from build123d import *

# Parameters (mm, degrees)
SKETCH1_W              = 44.45
SKETCH1_H              = 76.2
BOSS_EXTRUDE1_DEPTH    = 114.3
CUT_EXTRUDE1_REACH     = 124.516
SKETCH2_R              = 9.525
SKETCH3_W              = 22.86
SKETCH3_H              = 27.94
CUT_EXTRUDE2_DEPTH     = 19.05
CUT_EXTRUDE3_REACH     = 124.516
SKETCH4_W              = 34.925
SKETCH4_H              = 19.05
FILLET1_R              = 9.525
F_10_CLEARANCE_HOLE1_D = 5.1054
CUT_EXTRUDE4_REACH     = 130.421


with BuildPart() as part:
    # Sketch1 → Boss-Extrude1 (new body)
    with BuildSketch(Plane(origin=(0, 0, 0), x_dir=(0, 0, -1), z_dir=(1, 0, 0))):
        Rectangle(SKETCH1_W, SKETCH1_H)
    extrude(amount=BOSS_EXTRUDE1_DEPTH)

    # Sketch2 → Cut-Extrude1 (cut, up to next)
    with BuildSketch(Plane(origin=(114.3, 0, 0), x_dir=(0, 0, -1), z_dir=(1, 0, 0)), mode=Mode.PRIVATE) as cut_extrude1_sk1:
        with Locations((1.588, -4.0132)):
            Circle(SKETCH2_R)
    cut_extrude1_tool1 = extrude(cut_extrude1_sk1.sketch, amount=-CUT_EXTRUDE1_REACH, mode=Mode.PRIVATE) & part.part
    add(cut_extrude1_tool1.solids().sort_by_distance((114.3, -4.0132, -1.588))[0], mode=Mode.SUBTRACT)

    # Sketch3 → Cut-Extrude2 (cut)
    with BuildSketch(Plane.XY.offset(22.225)):
        with Locations((102.87, 24.13)):
            Rectangle(SKETCH3_W, SKETCH3_H)
    extrude(amount=-CUT_EXTRUDE2_DEPTH, mode=Mode.SUBTRACT)

    # Sketch4 → Cut-Extrude3 (cut, up to next)
    with BuildSketch(Plane(origin=(0, 0, 0), x_dir=(0, 0, -1), z_dir=(1, 0, 0)), mode=Mode.PRIVATE) as cut_extrude3_sk1:
        with Locations((4.7625, 28.575)):
            Rectangle(SKETCH4_W, SKETCH4_H)
    cut_extrude3_tool1 = extrude(cut_extrude3_sk1.sketch, amount=CUT_EXTRUDE3_REACH, mode=Mode.PRIVATE) & part.part
    add(cut_extrude3_tool1.solids().sort_by_distance((0, 28.575, -4.7625))[0], mode=Mode.SUBTRACT)

    # Fillet1
    fillet1_edges = [part.edges().sort_by_distance(p)[0] for p in [
        (91.44, 14.605, 3.175),
    ]]
    fillet(fillet1_edges, radius=FILLET1_R)

    # #10 Clearance Hole1 (through all)
    with Locations(Plane(origin=(0, 0, -22.225), x_dir=(-1, 0, 0), z_dir=(0, 0, -1))):
        with Locations((-47.625, 28.6385), (-79.375, -31.8135), (-47.625, -31.8135), (-79.375, 28.6385)):
            Hole(F_10_CLEARANCE_HOLE1_D / 2)

    # Sketch9 → Cut-Extrude4 (cut, up to next)
    with BuildSketch(Plane.XY.offset(22.225), mode=Mode.PRIVATE) as cut_extrude4_sk1:
        with BuildLine():
            Line((50.1777, 28.6385), (50.1777, 26.0985))
            ThreePointArc((50.1777, 26.0985), (47.625, 23.5458), (45.0723, 26.0985))
            Line((45.0723, 26.0985), (45.0723, 28.6385))
            ThreePointArc((45.0723, 28.6385), (47.625, 31.1912), (50.1777, 28.6385))
        make_face()
    cut_extrude4_tool1 = extrude(cut_extrude4_sk1.sketch, amount=-CUT_EXTRUDE4_REACH, mode=Mode.PRIVATE) & part.part
    # Sketch9 → Cut-Extrude4 (cut, up to next)
    with BuildSketch(Plane.XY.offset(22.225), mode=Mode.PRIVATE) as cut_extrude4_sk2:
        with BuildLine():
            Line((81.9277, 28.6385), (81.9277, 26.0985))
            ThreePointArc((81.9277, 26.0985), (79.375, 23.5458), (76.8223, 26.0985))
            Line((76.8223, 26.0985), (76.8223, 28.6385))
            ThreePointArc((76.8223, 28.6385), (79.375, 31.1912), (81.9277, 28.6385))
        make_face()
    cut_extrude4_tool2 = extrude(cut_extrude4_sk2.sketch, amount=-CUT_EXTRUDE4_REACH, mode=Mode.PRIVATE) & part.part
    # Sketch9 → Cut-Extrude4 (cut, up to next)
    with BuildSketch(Plane.XY.offset(22.225), mode=Mode.PRIVATE) as cut_extrude4_sk3:
        with BuildLine():
            Line((81.9277, -31.8135), (81.9277, -34.3535))
            ThreePointArc((81.9277, -34.3535), (79.375, -36.9062), (76.8223, -34.3535))
            Line((76.8223, -34.3535), (76.8223, -31.8135))
            ThreePointArc((76.8223, -31.8135), (79.375, -29.2608), (81.9277, -31.8135))
        make_face()
    cut_extrude4_tool3 = extrude(cut_extrude4_sk3.sketch, amount=-CUT_EXTRUDE4_REACH, mode=Mode.PRIVATE) & part.part
    # Sketch9 → Cut-Extrude4 (cut, up to next)
    with BuildSketch(Plane.XY.offset(22.225), mode=Mode.PRIVATE) as cut_extrude4_sk4:
        with BuildLine():
            Line((50.1777, -31.8135), (50.1777, -34.3535))
            ThreePointArc((50.1777, -34.3535), (47.625, -36.9062), (45.0723, -34.3535))
            Line((45.0723, -34.3535), (45.0723, -31.8135))
            ThreePointArc((45.0723, -31.8135), (47.625, -29.2608), (50.1777, -31.8135))
        make_face()
    cut_extrude4_tool4 = extrude(cut_extrude4_sk4.sketch, amount=-CUT_EXTRUDE4_REACH, mode=Mode.PRIVATE) & part.part
    add(cut_extrude4_tool1.solids().sort_by_distance((47.625, 27.3685, 22.225))[0], mode=Mode.SUBTRACT)
    add(cut_extrude4_tool2.solids().sort_by_distance((79.375, 27.3685, 22.225))[0], mode=Mode.SUBTRACT)
    add(cut_extrude4_tool3.solids().sort_by_distance((79.375, -33.0835, 22.225))[0], mode=Mode.SUBTRACT)
    add(cut_extrude4_tool4.solids().sort_by_distance((47.625, -33.0835, 22.225))[0], mode=Mode.SUBTRACT)


solid = part.part
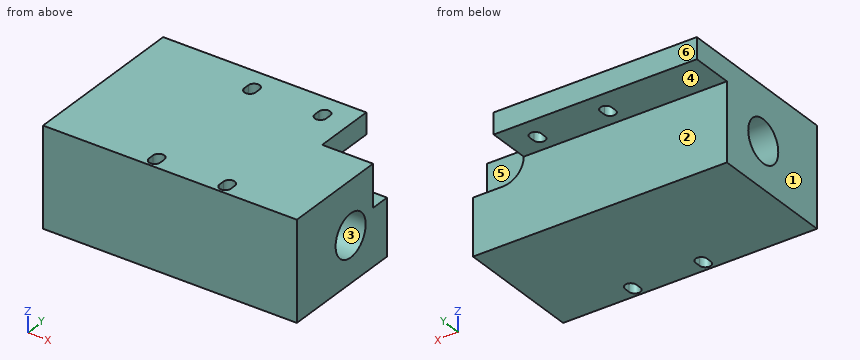
Geometry check sheet. Reference: the model listing, model coordinates, mm. Face numbers are marked on the shaded views. A direction names the side the tool comes from. Give positions to 0.01 mm unless a question says otherwise; leave off trailing zeros. Loops run counter-clockwise (first coordinate to the right, second up) from the corner with the lowest first, then second, coordinate; pieces in that order, holes last. Notation, with made-up numbers: M -1.75,-35.75 L 33.25,-35.75 A24 cw 33.25,-13.75 Z; hole C 24.25,79.5 d7. An arc over 180 degrees is marked long. Write each question's results on one line, items separated by ' | '.
1) Section check B-B, the plane y = -30.5. Record the boundary of the cut face in (x, z) (3 decimals), plus the area to 3 significant figures.
Answers follow:
outline: M 0,-22.225 L 45.436,-22.225 L 45.436,22.225 L 0,22.225 Z; M 49.814,-22.225 L 77.186,-22.225 L 77.186,22.225 L 49.814,22.225 Z; M 81.564,-22.225 L 114.3,-22.225 L 114.3,22.225 L 81.564,22.225 Z | area: 4,690 mm2
2) Section check A-A, the plane z = 4.5. Count the separate pieces of the cut face and the enclosed holes in it, plus the area to 3 significant figures.
Answers follow:
separate pieces: 2 | enclosed holes: 2 | area: 4,630 mm2
3) Gauge pin test, flat ends, axial feed: pin 1 (17 mm diameter, centred on y = -4.01, z = -1.59, fed in from -X); pin 2 (1.3 mm diameter, centred on y = 27, z = 18.5, fed in from +X); pin 3 (8 mm diameter, centred on x = 59, z = 5.5, fed in from +Y); pin 4 (2.5 mm diameter, centred on x = 105.5, y = 16, fed in from +Z) (3 decimals). Record the tip position at first contact, or that the pin passes through.
Answers follow:
pin 1: through | pin 2: x = 91.44 | pin 3: y = 19.05 | pin 4: z = 3.175
4) Release check for a two-part mould opening along Y. For the marked faces 1, 2 and 3 record: +Y half, -Y half, draft (parallel to the pull), parting line (faces both ways), or undercut.
Answers follow:
face 1: draft | face 2: +Y half | face 3: undercut
5) Tool access check on the marked faces 4, 5 and 6. Record the directions out of +Z, -Z, +X, -X, +Y, -Y that give a thin tool (end or side, any length) a straight path to the whole face; none if there is none.
Answers follow:
face 4: -Z, +X, -X, +Y | face 5: +Z, +X, +Y | face 6: +Z, -Z, +X, -X, +Y
6) Thickness scan on line 1 (Y direction, x = 81.5, z = 15); line 2 (Z direction, x = 20.5, y = 33) (3 decimals); line 3 (Y direction, x = 89, z = 9). Record the ranges inside material, lowest first.
Answers follow:
line 1: -38.1 to -35.77, -30.4 to 24.68, 30.05 to 38.1 | line 2: 12.7 to 22.225 | line 3: -38.1 to 19.05
7) Section check D-D, the plane y = 1. Record the boundary of the cut face in (x, z) (3 decimals).
Answers follow:
outline: M 0,-22.225 L 114.3,-22.225 L 114.3,-9.687 L 0,-9.687 Z; M 0,6.511 L 114.3,6.511 L 114.3,22.225 L 0,22.225 Z
